```python
from build123d import *

# Parameters (mm, degrees)
SKETCH1_R           = 25
BOSS_EXTRUDE1_DEPTH = 52
SKETCH2_R           = 12
BOSS_EXTRUDE2_DEPTH = 15
SKETCH3_R           = 25
BOSS_EXTRUDE3_DEPTH = 3
FILLET1_R           = 10
FILLET2_R           = 10
SKETCH4_R           = 20
CUT_EXTRUDE1_DEPTH  = 18


with BuildPart() as part:
    # Sketch1 → Boss-Extrude1 (new body)
    with BuildSketch(Plane(origin=(0, 0, 0), x_dir=(1, 0, 0), z_dir=(0, 1, 0))):
        with Locations(Location((0, 0, 0), (0, 0, 90))):
            Circle(SKETCH1_R)
    extrude(amount=BOSS_EXTRUDE1_DEPTH)

    # Sketch2 → Boss-Extrude2 (add)
    with BuildSketch(Plane(origin=(0, 52, 0), x_dir=(1, 0, 0), z_dir=(0, 1, 0))):
        with Locations(Location((0, 0, 0), (0, 0, 270))):
            Circle(SKETCH2_R)
    extrude(amount=BOSS_EXTRUDE2_DEPTH)

    # Sketch3 → Boss-Extrude3 (add)
    with BuildSketch(Plane(origin=(0, 67, 0), x_dir=(1, 0, 0), z_dir=(0, 1, 0))):
        with Locations(Location((0, 0, 0), (0, 0, 90))):
            Circle(SKETCH3_R)
    extrude(amount=BOSS_EXTRUDE3_DEPTH)

    # Fillet1
    fillet1_edges = [part.edges().sort_by_distance(p)[0] for p in [
        (0, 52, -12),
    ]]
    fillet(fillet1_edges, radius=FILLET1_R)

    # Fillet2
    # the kernel refuses this fillet: 10 mm, written as the material it adds along each edge
    with BuildSketch(Plane(origin=(0, 67, 0), x_dir=(0, 0, 1), z_dir=(-1, 0, 0))) as fillet2_piece_1:
        with BuildLine():
            CenterArc((20.660254038, -10), FILLET2_R, 90, 60)
            Line((20.660254038, 0), (20.660254038, 0.2))
            Line((20.660254038, 0.2), (12, 0.2))
            Line((12, 0.2), (11.8, 0))
            ThreePointArc((11.8, 0), (11.8, -2.5), (11.826794919, -4.9))
            Line((11.826794919, -4.9), (12, -5))
        make_face()
    revolve(axis=Axis((0, 67, 0), (0, 1, 0)))

    # Sketch4 → Cut-Extrude1 (cut)
    with BuildSketch(Plane(origin=(0, 0, 0), x_dir=(-1, 0, 0), z_dir=(0, -1, 0))):
        with Locations(Location((0, 0, 0), (0, 0, 90))):
            Circle(SKETCH4_R)
    extrude(amount=-CUT_EXTRUDE1_DEPTH, mode=Mode.SUBTRACT)


solid = part.part
```
CAD build for the part. Positions are in the model's coordinates, mm. A direction names the side the tool comes from. Give positions to 0.01 mm unless a question says otherwise; leave off trailing zeros. Loops run counter-clockwise (first coordinate to the right, second up) from the corner with the lowest first, then second, coordinate; pieces in that order, holes last. Notation, with made-up numbers: (-12, 26) - (39, 26) arc R13 ccw to (39, 40) - close; hole circle Ø9 at (35.25, -21). An arc over 180 degrees is marked (long way). Put each result on its own line as item: value.
Q1. Slice it at A-A (z = 0). Give the cut face in (x, y).
Filled in:
outline: (-25, 0) - (-20, 0) - (-20, 18) - (20, 18) - (20, 0) - (25, 0) - (25, 52) - (22, 52) arc R10 cw to (12, 62) arc R10 cw to (20.66, 67) - (25, 67) - (25, 70) - (-25, 70) - (-25, 67) - (-20.66, 67) arc R10 cw to (-12, 62) arc R10 cw to (-22, 52) - (-25, 52) - close
Q2. Tool access for faces 1 (the face through (0, 18, 0)), 2 (the face through (-19, 67, 9)), 3 (the face through (0, 70, 0)): list every direction of +Z, -Z, +X, -X, +Y, -Y with a clear straight run to the whole face (end or side of a thin tool).
Filled in:
face 1: -Y
face 2: none
face 3: +Z, -Z, +X, -X, +Y
Q3. Mould opens along Z. For faces 4 (the face through (-7.509, 68.479, -23.846)), 5 (the face through (22.1, 52, -1.7)), 6 (the face through (-19.524, 8.874, 4.336)) say: pulls with the +Z half, pulls with the -Z half, needs draft (parallel to the pull), parting line crosses it, or undercut.
Filled in:
face 4: parting line crosses it
face 5: needs draft
face 6: undercut
Q4. Slice it at C-C (y = 14.5). Give the cut face in (x, z), plus the area to 3 significant figures.
Filled in:
outline: circle Ø50 at (0, 0); hole circle Ø40 at (0, 0)
area: 707 mm²
Q5. Slice it at B-B (x = 0). Give the cut face in (y, z).
Filled in:
outline: (0, -25) - (52, -25) - (52, -22) arc R10 cw to (62, -12) arc R10 cw to (67, -20.66) - (67, -25) - (70, -25) - (70, 25) - (67, 25) - (67, 20.66) arc R10 cw to (62, 12) arc R10 cw to (52, 22) - (52, 25) - (0, 25) - (0, 20) - (18, 20) - (18, -20) - (0, -20) - close
Q6. Flat gauge pins, fed straight in: pin 1 (2 mm diameter, centred on y = 36, z = 17, fed in from -X); pin 2 (6 mm diameter, centred on y = 34, z = -8, fed in from +X); pin 3 (2 mm diameter, centred on y = 46.5, z = -15, fed in from -X). Where does each tip first touch, or does it go through?
Filled in:
pin 1: stops at x = -19.21
pin 2: stops at x = 24.49
pin 3: stops at x = -20.71
Q7. Probe line 1 along Y through (x, z) = (-8, -23); line 2 along X through (y, z) = (11.25, 0); line 3 along Y through (x, z) = (4, 10). List the from-to ranges inside material, lowest first.
Filled in:
line 1: y = 0 to 52, 67 to 70
line 2: x = -25 to -20, 20 to 25
line 3: y = 18 to 70
Q8. Slice it at D-D (y = 36). Give the cut face in (x, z).
Filled in:
outline: circle Ø50 at (0, 0)
